Could you check a few things on this model? Use its own coordinates, in mm. A direction names the side the tool comes from. Coordinates: 2 decimals unless noted, no trailing zeros. Order: outer loops, then holes, each group sorted by start corner. A loop starts at its lowest first (then second) coordinate and runs counter-clockwise, first axis right, second up. Notation, with made-up numbers: (-2.75, 76.5) -> (28.25, 76.5) arc R21 ccw to (28.25, 101.5) -> close; hole circle Ø3 at (-10.75, 52.25). An arc over 180 degrees is marked (long way). Use a Markdown table: item, result. Add a question column.
1) Which directions (+Z, -Z, +X, -X, +Y, -Y) give clear straight access to the entire face, cutting with the end or side of a thin tool? Please do faces 4 (the cylindrical face through (-47.954, -21.86, -2.11)), 5 (the flat face through (-41.2, 8, -25.2)), 6 (the flat face through (-10, 0, -1)).
2) If we section it at A-A (y = -3): Write out the boundary of the cut face in (x, z), plus the area to 3 significant figures.
3) Will these pins go through, and if not, where does the flat tip stop? pin 1 Ø8 at (y, z) = (-19.5, -37) entering from +X; pin 2 Ø10 at (x, y) = (-2, -9.5) entering from +Z; pin 3 Ø1 at (x, y) = (10.5, -10.5) entering from -Z.
4) Thinking about a two-plate mould opening in Z: for faces 1 (the flat face through (10, -12, -1)), 2 (the cylindrical face through (51.73, -12.28, 21.45)), 3 (the flat face through (41.2, -32, -25.2)), which applies, +Z half, -Z half, draft (parallel to the pull), parting line (faces both ways), or undercut?
5) If I drill on L1, parallel to Z at x = 0, y = -21; L2, parallel to Z at x = 0, y = -3.5, over which ranges is the centre line in solid material (lowest first)? Write a range as [from, to].
6) If we section it at D-D (y = -17): Write out the boundary of the cut face in (x, z), plus the area to 3 significant figures.
7) If we section it at C-C (z = -24): Write out the boundary of the cut face in (x, y), plus the area to 3 significant figures.
8) If we section it at B-B (x = -25): Write out the boundary of the cut face in (y, z), plus the area to 3 significant figures.
```python
from build123d import *

# Parameters (mm, degrees)
SKETCH3_R                       = 1
HOLE_FOR_SCREW_BLADE_CASE_DEPTH = 100


with BuildPart() as part:
    # Sketch2 → Blade Casing Revolve (revolve)
    with BuildSketch(Plane.XY):
        Polygon((0, 0), (48, 0), (48, 8), (56, 8), (56, -32), (48, -32), (48, -12), (0, -12), align=None)
    revolve(axis=Axis((0, -12, 0), (0, 1, 0)))

    # Sketch3 → Hole for Screw (Blade Case) (cut)
    with BuildSketch(Plane(origin=(0, 0, 0), x_dir=(1, 0, 0), z_dir=(0, 1, 0))):
        with Locations(Location((0, 0, 0), (0, 0, 180))):
            Circle(SKETCH3_R)
    extrude(amount=-HOLE_FOR_SCREW_BLADE_CASE_DEPTH, mode=Mode.SUBTRACT)


solid = part.part
```
Answer sheet:
| question | item | result |
|---|---|---|
| 1 | face 4 | -Y |
| 1 | face 5 | +Z, -Z, +X, -X, +Y |
| 1 | face 6 | +Y |
| 2 | outline | circle Ø112 at (0, 0); hole circle Ø2 at (0, 0) |
| 2 | area | 9,850 mm2 |
| 3 | pin 1 | x = 45.24 |
| 3 | pin 2 | z = 56 |
| 3 | pin 3 | z = -55.1 |
| 4 | face 1 | undercut |
| 4 | face 2 | parting line |
| 4 | face 3 | draft |
| 5 | L1 | [-56, -48], [48, 56] |
| 5 | L2 | [-56, -1], [1, 56] |
| 6 | outline | circle Ø112 at (0, 0); hole circle Ø96 at (0, 0) |
| 6 | area | 2,610 mm2 |
| 7 | outline | (-50.6, -32) -> (-41.57, -32) -> (-41.57, -12) -> (41.57, -12) -> (41.57, -32) -> (50.6, -32) -> (50.6, 8) -> (41.57, 8) -> (41.57, 0) -> (-41.57, 0) -> (-41.57, 8) -> (-50.6, 8) -> close |
| 7 | area | 1,720 mm2 |
| 8 | outline | (-32, -50.11) -> (8, -50.11) -> (8, -40.98) -> (0, -40.98) -> (0, 40.98) -> (8, 40.98) -> (8, 50.11) -> (-32, 50.11) -> (-32, 40.98) -> (-12, 40.98) -> (-12, -40.98) -> (-32, -40.98) -> close |
| 8 | area | 1,710 mm2 |
